from build123d import *

# Parameters (mm, degrees)
F0_R     = 3.9751
F1_DEPTH = 25.4
F2_R     = 3.9751
F2_R_2   = 3.175
F3_DEPTH = 2.54
F4_R     = 3.9751
F4_R_2   = 3.175
F5_DEPTH = 2.54


with BuildPart() as f1:
    # F0 (on Front) → F1 (new body)
    with BuildSketch(Plane.XZ):
        Circle(F0_R)
    extrude(amount=F1_DEPTH)

    # F2 (on face) → F3 (cut)
    with BuildSketch(Plane.XZ.offset(25.4)):
        Circle(F2_R)
        Circle(F2_R_2, mode=Mode.SUBTRACT)
    extrude(amount=-F3_DEPTH, mode=Mode.SUBTRACT)

    # F4 (on Front) → F5 (cut)
    with BuildSketch(Plane.XZ):
        Circle(F4_R)
        Circle(F4_R_2, mode=Mode.SUBTRACT)
    extrude(amount=F5_DEPTH, mode=Mode.SUBTRACT)


solid = f1.part
For this review, take the finished solid that the model builds, in its own axes (mm). A direction names the side the tool comes from. Give positions to 0.01 mm unless a question says otherwise; leave off trailing zeros. Loops run counter-clockwise (first coordinate to the right, second up) from the corner with the lowest first, then second, coordinate; pieces in that order, holes last.
Item 1: Take a section at B-B, the plane z = 0. State the section outline as (x, y) points (3 decimals).
Item 2: Take a section at A-A, the plane x = 0. State the section outline as (y, z) points (3 decimals).
Item 3: Tool access review of faces 1 (the flat face through (-3, -22.86, -2)), 2 (the flat face through (-3, -2.54, -2)), 3 (the flat face through (0, 0, 0)): name each direction out of +Z, -Z, +X, -X, +Y, -Y from which nothing blocks a thin tool from reaching the whole face with its end or side.
Item 4: For line 1 along Z through (x, y) = (0, -24) (3 decimals); line 2 along Y through (x, z) = (-1.5, -3.5); line 3 along Z through (x, y) = (3.5, -4), list the stretches that pass through material, from the lowest coordinate up.
Item 5: Take a section at D-D, the plane x = 3.5. State the section outline as (y, z) points, and give its area (3 significant figures).
Item 6: Insertion check: pin 1 (1.5 mm diameter, centred on x = -1, z = 1, fed in from +Y); pin 2 (2 mm diameter, centred on x = 3, y = -10.5, fed in from -Z); pin 3 (1.5 mm diameter, centred on y = -4.5, z = -1, fed in from -X). Each pin has a flat end and moves straight along its axis. Give the tip position at first contact, or say it passes through.
Item 7: Take a section at C-C, the plane y = -10. State the section outline as (x, z) points, and give its area (3 significant figures).
Calculated:
1. outline: (-3.975, -22.86) - (-3.175, -22.86) - (-3.175, -25.4) - (3.175, -25.4) - (3.175, -22.86) - (3.975, -22.86) - (3.975, -2.54) - (3.175, -2.54) - (3.175, 0) - (-3.175, 0) - (-3.175, -2.54) - (-3.975, -2.54) - close
2. outline: (-25.4, -3.175) - (-22.86, -3.175) - (-22.86, -3.975) - (-2.54, -3.975) - (-2.54, -3.175) - (0, -3.175) - (0, 3.175) - (-2.54, 3.175) - (-2.54, 3.975) - (-22.86, 3.975) - (-22.86, 3.175) - (-25.4, 3.175) - close
3. face 1: -Y
3. face 2: +Y
3. face 3: +Z, -Z, +X, -X, +Y
4. line 1: z = -3.175 to 3.175
4. line 2: y = -22.86 to -2.54
4. line 3: z = -1.88 to 1.88
5. outline: (-22.86, -1.88) - (-2.54, -1.88) - (-2.54, 1.88) - (-22.86, 1.88) - close
5. area: 76.6 mm2
6. pin 1: stops at y = 0
6. pin 2: stops at z = -3.44
6. pin 3: stops at x = -3.97
7. outline: circle Ø7.95 at (0, 0)
7. area: 49.6 mm2
